Input: dimensioned drawing with shaded views. Units: mm. Origin: part minimum x, y, z. A direction names the side the tool comes from. Give positions to 0.01 mm unless a question says otherwise; leave off trailing zeros. Loops run counter-clockwise (first coordinate to the right, second up) from the corner with the lowest first, then second, coordinate; pieces in that order, holes last. Notation, with made-up numbers: (88, -31) -> (115, -31) arc R22 cw to (115, -22) -> close; hole circle Ø2 at (31.25, 84). An arc over 180 degrees is marked (long way). Answer as a JSON object with one key per item and string values.
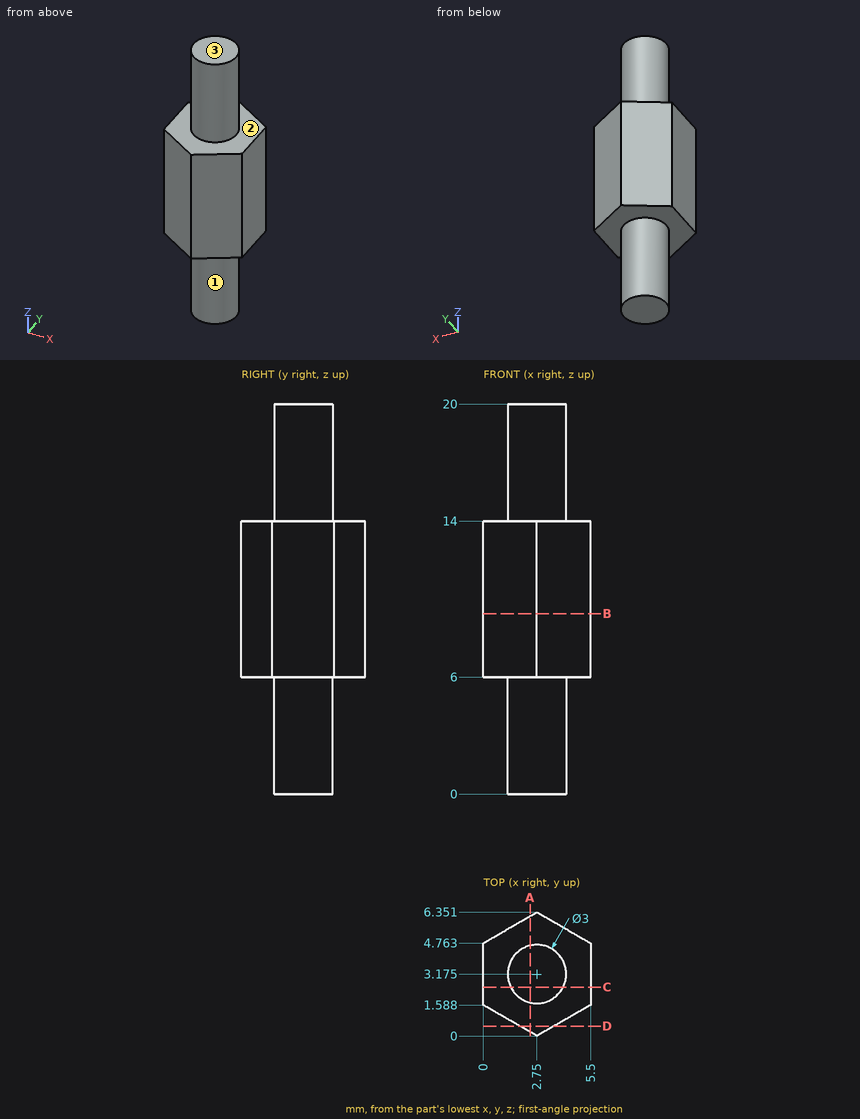
Q1. Section C-C, the plane y = 2.5. Return the cut outline in (x, z).
Evaluation:
{"outline": "(0, 6) -> (1.41, 6) -> (1.41, 0) -> (4.09, 0) -> (4.09, 6) -> (5.5, 6) -> (5.5, 14) -> (4.09, 14) -> (4.09, 20) -> (1.41, 20) -> (1.41, 14) -> (0, 14) -> close"}
Q2. Pin query (flat end, axial travel): pin 1 (1.5 mm diameter, centred on y = 0.5, z = 9.5, fed in from +X) (1 decimal). Return the tip coordinate at first contact, or that it passes through.
Evaluation:
{"pin 1": "stops at x = 4.9"}
Q3. Ray query, line 1 along X through (y, z) = (3.25, 19); line 2 along Z through (x, y) = (4.75, 2.25); line 3 along Y through (x, z) = (5, 7). Return the intervals inside material, ascending.
Evaluation:
{"line 1": "x = 1.25 to 4.25", "line 2": "z = 6 to 14", "line 3": "y = 1.3 to 5.05"}
Q4. Section D-D, the plane y = 0.5. Return the cut outline in (x, z).
Evaluation:
{"outline": "(1.88, 6) -> (3.62, 6) -> (3.62, 14) -> (1.88, 14) -> close"}
Q5. Section B-B, the plane z = 9.25. Return the cut outline in (x, y), then the cut area to 3 significant figures.
Evaluation:
{"outline": "(0, 1.59) -> (2.75, 0) -> (5.5, 1.59) -> (5.5, 4.76) -> (2.75, 6.35) -> (0, 4.76) -> close", "area": "26.2 mm2"}
Q6. Access query for the marked faces 1, 2 and 3. Directions: +Z, -Z, +X, -X, +Y, -Y. A direction counts if a zero-diameter tool reaches every point of the face in a straight line with its end or side. Return the directions, or none.
Evaluation:
{"face 1": "-Z", "face 2": "+Z", "face 3": "+Z, +X, -X, +Y, -Y"}
Q7. Section A-A, the plane x = 2.4. Return the cut outline in (y, z).
Evaluation:
{"outline": "(0.2, 6) -> (1.72, 6) -> (1.72, 0) -> (4.63, 0) -> (4.63, 6) -> (6.15, 6) -> (6.15, 14) -> (4.63, 14) -> (4.63, 20) -> (1.72, 20) -> (1.72, 14) -> (0.2, 14) -> close"}
